Check sheet for the modelled part. Datum: model origin and axes. Units: mm. A direction names the side the tool comes from. Give positions to 0.01 mm unless a question says otherwise; leave off trailing zeros. Write each loop counter-clockwise with the first axis right and the second up, starting at its lowest first coordinate (ties: lowest second). Pieces come first, ordered by that corner, then holes. Notation, with made-up numbers: (-32.5, 58.25) -> (-23.5, 58.25) arc R14 ccw to (-23.5, 62.25) -> close; hole circle Ø8 at (72.5, 89.5). An arc over 180 degrees is marked (long way). Answer as a JSON object with one key per item and string values.
from build123d import *

# Parameters (mm, degrees)
SKETCH1_R               = 4.5
SKETCH1_R_2             = 2.5
BOSS_EXTRUDE1_DEPTH     = 2.5
SKETCH2_R               = 15
BOSS_EXTRUDE2_DEPTH     = 2
SKETCH3_R               = 2.159
CUT_EXTRUDE1_DEPTH      = 1
CUT_EXTRUDE1_DEPTH_BACK = 5.5
FILLET2_R               = 0.508


with BuildPart() as part:
    # Sketch1 → Boss-Extrude1 (new body)
    with BuildSketch(Plane.XY):
        Circle(SKETCH1_R)
        Circle(SKETCH1_R_2, mode=Mode.SUBTRACT)
    extrude(amount=BOSS_EXTRUDE1_DEPTH)

    # Sketch2 → Boss-Extrude2 (add)
    with BuildSketch(Plane.XY.offset(2.5)):
        Circle(SKETCH2_R)
    extrude(amount=BOSS_EXTRUDE2_DEPTH)

    # Sketch3 → Cut-Extrude1 (cut, two sides)
    with BuildSketch(Plane.XY.offset(4.5)) as cut_extrude1_sk:
        with Locations((-9.525, 0)):
            Circle(SKETCH3_R)
        with Locations((9.525, 0)):
            Circle(SKETCH3_R)
    extrude(amount=CUT_EXTRUDE1_DEPTH, mode=Mode.SUBTRACT)
    extrude(cut_extrude1_sk.sketch, amount=-CUT_EXTRUDE1_DEPTH_BACK, mode=Mode.SUBTRACT)

    # Fillet2
    fillet2_edges = [part.edges().sort_by_distance(p)[0] for p in [
        (-15, 0, 4.5),
        (-15, 0, 2.5),
    ]]
    fillet(fillet2_edges, radius=FILLET2_R)


solid = part.part
1. Sectioned sample at B-B, the plane z = 2.15. Enter the section's corners in (x, y), plus the area to 3 significant figures.
Determined:
{"outline": "circle Ø9 at (0, 0); hole circle Ø5 at (0, 0)", "area": "44.0 mm^2"}
2. Scan lines: L1, parallel to Y at x = 0, z = 1.45; L2, parallel to Z at x = 7, y = 10; L3, parallel to Y at x = -11, z = 3.8. Record each from-to range of solid material in increasing order. Write a range as [from, to].
Determined:
{"L1": "[-4.5, -2.5], [2.5, 4.5]", "L2": "[2.5, 4.5]", "L3": "[-10.2, -1.58], [1.58, 10.2]"}
3. Sectioned sample at A-A, the plane y = 0. Enter the section's corners in (x, z).
Determined:
{"outline": "(-15, 3.01) arc R0.51 ccw to (-14.49, 2.5) -> (-11.68, 2.5) -> (-11.68, 4.5) -> (-14.49, 4.5) arc R0.51 ccw to (-15, 3.99) -> close; (-7.37, 2.5) -> (-4.5, 2.5) -> (-4.5, 0) -> (-2.5, 0) -> (-2.5, 2.5) -> (2.5, 2.5) -> (2.5, 0) -> (4.5, 0) -> (4.5, 2.5) -> (7.37, 2.5) -> (7.37, 4.5) -> (-7.37, 4.5) -> close; (11.68, 2.5) -> (14.49, 2.5) arc R0.51 ccw to (15, 3.01) -> (15, 3.99) arc R0.51 ccw to (14.49, 4.5) -> (11.68, 4.5) -> close"}
4. Go/stop test with flat-tipped pins: P1, Ø4.5, axis at x = 0, y = 0, coming from the -Z side; P2, Ø1.5, axis at y = -5.5, z = 1.5, coming from the -X side; P3, Ø14.5, axis at x = 1.5, y = -6, coming from the -Z side; P4, Ø1.5, axis at y = 4, z = 2, coming from the -X side. Record where each tip stops, or that it passes through.
Determined:
{"P1": "z = 2.5", "P2": "through", "P3": "z = 0", "P4": "x = -14.42"}
5. Access from +Z, -Z, +X, -X, +Y, -Y to the whole of each face (thin tool, end or side, straight path). Record for faces 4 (the face through (-3.4, 3.4, 2.5)), 5 (the face through (7.368, 0.095, 3.514)).
Determined:
{"face 4": "-Z", "face 5": "+Z, -Z"}
6. Mould release check, pull along Y, two halves, no side actions. Record for faces 1 (the face through (-0.54, -2.44, 1.23)), 2 (the face through (0, 0, 4.5)), 3 (the face through (-14.985, 0.66, 3.493)): released by +Y, released by -Y, zero draft, split by the parting line, or undercut.
Determined:
{"face 1": "undercut", "face 2": "zero draft", "face 3": "split by the parting line"}
7. Sectioned sample at C-C, the plane x = 0. Enter the section's corners in (y, z).
Determined:
{"outline": "(-15, 3.01) arc R0.51 ccw to (-14.49, 2.5) -> (-4.5, 2.5) -> (-4.5, 0) -> (-2.5, 0) -> (-2.5, 2.5) -> (2.5, 2.5) -> (2.5, 0) -> (4.5, 0) -> (4.5, 2.5) -> (14.49, 2.5) arc R0.51 ccw to (15, 3.01) -> (15, 3.99) arc R0.51 ccw to (14.49, 4.5) -> (-14.49, 4.5) arc R0.51 ccw to (-15, 3.99) -> close"}
